from build123d import *

# Parameters (mm, degrees)
SKETCH1_W           = 46.3
SKETCH1_H           = 189.86
SKETCH1_R           = 10.5
SKETCH1_R_2         = 8
SKETCH1_R_3         = 1.5
BOSS_EXTRUDE1_DEPTH = 3
FILLET1_R           = 25


with BuildPart() as part:
    # Sketch1 → Boss-Extrude1 (new body)
    # profile 1 of 2: a face of its own
    with BuildSketch(Plane.XY):
        Rectangle(SKETCH1_W, SKETCH1_H)
        with Locations((0, 71.93)):
            Circle(SKETCH1_R, mode=Mode.SUBTRACT)
        with Locations((0, -78.93)):
            Circle(SKETCH1_R_2, mode=Mode.SUBTRACT)
    # profile 2 of 2: a face of its own
    with BuildSketch(Plane.XY):
        with Locations((0, 71.93)):
            Circle(SKETCH1_R)
        with Locations((0, 78.93)):
            Circle(SKETCH1_R_3, mode=Mode.SUBTRACT)
        with Locations((7, 71.93)):
            Circle(SKETCH1_R_3, mode=Mode.SUBTRACT)
        with Locations((0, 64.93)):
            Circle(SKETCH1_R_3, mode=Mode.SUBTRACT)
        with Locations((-7, 71.93)):
            Circle(SKETCH1_R_3, mode=Mode.SUBTRACT)
        with Locations((0, 71.93)):
            Circle(SKETCH1_R_3, mode=Mode.SUBTRACT)
    extrude(amount=BOSS_EXTRUDE1_DEPTH)

    # Fillet1
    # the kernel refuses this fillet: 25 mm, written as the material it takes off along each edge
    with BuildSketch(Plane(origin=(-23.15, -94.93, -62.5), x_dir=(0, 1, 0), z_dir=(0, 0, 1)), Plane(origin=(23.15, -94.93, -62.5), x_dir=(-1, 0, 0), z_dir=(0, 0, 1))) as fillet1_piece_1:
        with BuildLine():
            CenterArc((FILLET1_R, -FILLET1_R), FILLET1_R, 90, 90)
            Line((0, -FILLET1_R), (0, 0))
            Line((0, 0), (FILLET1_R, 0))
        make_face()
    extrude(amount=128, mode=Mode.SUBTRACT)
    with BuildSketch(Plane(origin=(-23.15, 94.93, -62.5), x_dir=(0, -1, 0), z_dir=(0, 0, 1)), Plane(origin=(23.15, 94.93, -62.5), x_dir=(-1, 0, 0), z_dir=(0, 0, 1))) as fillet1_piece_2:
        with BuildLine():
            CenterArc((FILLET1_R, FILLET1_R), FILLET1_R, 180, 90)
            Line((0, FILLET1_R), (0, 0))
            Line((0, 0), (FILLET1_R, 0))
        make_face()
    extrude(amount=128, mode=Mode.SUBTRACT)


solid = part.part
Input: part model. Units: mm. Frame: model coordinates. Coordinates: 2 decimals unless noted, no trailing zeros. Loops run counter-clockwise (first coordinate to the right, second up) from the corner with the lowest first, then second, coordinate; pieces in that order, holes last. Notation, with made-up numbers: (-26.75, 3) - (-18.75, 3) arc R18 ccw to (-18.75, 16) - close; hole circle Ø3 at (-21.5, -27). An arc over 180 degrees is marked (long way). Answer in a Markdown table with one row per item. Add a question column.
Item 1: Line query: line 1 along Y through (x, z) = (-1, 0.5); line 2 along X through (y, z) = (71.93, 1); line 3 along X through (y, z) = (-74.5, 0.4). Output: solid intervals per line, ascending. Write a range as [from, to].
Item 2: Section query C-C on x = -15. Return the cut outline in (y, z).
Item 3: Section query B-B on y = -78.93. Return the cut outline in (x, z), then the cut area to 3 significant figures.
Item 4: Contact query for flat-ended pins moving along their axis: P1, Ø1.8, axis at x = 0, y = 78.93, coming from the +Z side; P2, Ø1.5, axis at x = 1, z = 1, coming from the -Y side. Output: stop coordinate, or through.
Item 5: Mould query, pull axis Y, two halves, no side actions, for faces 1 (the cylindrical face through (-16.291, 87.132, 1.479)), 2 (the flat face through (0, 1, 3)), 3 (the cylindrical face through (-0.195, 80.417, 1.479)). Classes: released by +Y, released by -Y, zero draft, split by the parting line, or undercut.
Item 6: Section query A-A on z = 0.45. Return the cut outline in (x, y).
Recorded:
| question | item | result |
|---|---|---|
| 1 | line 1 | [-94.77, -86.87], [-70.99, 63.81], [66.05, 70.81], [73.05, 77.81], [80.05, 94.77] |
| 1 | line 2 | [-23.07, -8.5], [-5.5, -1.5], [1.5, 5.5], [8.5, 23.07] |
| 1 | line 3 | [-22.73, -6.66], [6.66, 22.73] |
| 2 | outline | (-88.4, 0) - (88.4, 0) - (88.4, 3) - (-88.4, 3) - close |
| 3 | outline | (-21.47, 0) - (-8, 0) - (-8, 3) - (-21.47, 3) - close; (8, 0) - (21.47, 0) - (21.47, 3) - (8, 3) - close |
| 3 | area | 80.8 mm^2 |
| 4 | P1 | through |
| 4 | P2 | y = -94.84 |
| 5 | face 1 | released by +Y |
| 5 | face 2 | zero draft |
| 5 | face 3 | undercut |
| 6 | outline | (-23.15, -69.93) arc R25 ccw to (0, -94.86) arc R25 ccw to (23.15, -69.93) - (23.15, 69.93) arc R25 ccw to (0, 94.86) arc R25 ccw to (-23.15, 69.93) - close; hole circle Ø3 at (-7, 71.93); hole circle Ø16 at (0, -78.93); hole circle Ø3 at (0, 64.93); hole circle Ø3 at (0, 71.93); hole circle Ø3 at (0, 78.93); hole circle Ø3 at (7, 71.93) |
